```python
from build123d import *

# Parameters (mm, degrees)
SKETCH_1_W          = 60
SKETCH_1_H          = 24
EXTRUDE_1_DEPTH     = 5
SKETCH_2_W          = 31.5
SKETCH_2_H          = 9
SKETCH_2_H_2        = 3
EXTRUDE_2_DEPTH     = 15
SKETCH_3_R          = 1.9
CUT_EXTRUDE_1_DEPTH = 24
SKETCH_4_R          = 4.5
CUT_EXTRUDE_2_DEPTH = 24
FILLET_1_R          = 10
CUT_EXTRUDE_3_DEPTH = 3
SKETCH_7_R          = 1.5
CUT_EXTRUDE_4_DEPTH = 3
CUT_EXTRUDE_5_DEPTH = 6
SKETCH_9_W          = 4.8
SKETCH_9_H          = 12.477545801
CUT_EXTRUDE_6_DEPTH = 3
SKETCH_10_W         = 4.8
SKETCH_10_H         = 29.172350056
CUT_EXTRUDE_7_DEPTH = 3
CHAMFER_1_SIZE      = 3


with BuildPart() as part:
    # Эскиз1 → Бобышка-Вытянуть1 (new body)
    with BuildSketch(Plane(origin=(0, 0, 0), x_dir=(1, 0, 0), z_dir=(0, 1, 0))):
        with Locations((30, 12)):
            Rectangle(SKETCH_1_W, SKETCH_1_H)
    extrude(amount=EXTRUDE_1_DEPTH)

    # Эскиз2 → Бобышка-Вытянуть2 (add)
    with BuildSketch(Plane(origin=(0, 5, 0), x_dir=(1, 0, 0), z_dir=(0, 1, 0))):
        with Locations((30, 4.5)):
            Rectangle(SKETCH_2_W, SKETCH_2_H)
        with Locations((30, 22.5)):
            Rectangle(SKETCH_2_W, SKETCH_2_H_2)
    extrude(amount=EXTRUDE_2_DEPTH)

    # Эскиз3 → Вырез-Вытянуть1 (cut)
    with BuildSketch(Plane.XY):
        with Locations((26.25, 15)):
            Circle(SKETCH_3_R)
    extrude(amount=-CUT_EXTRUDE_1_DEPTH, mode=Mode.SUBTRACT)

    # Эскиз4 → Вырез-Вытянуть2 (cut)
    with BuildSketch(Plane.XZ):
        with Locations(Location((7, -12, 0), (0, 0, 270))):
            Circle(SKETCH_4_R)
        with Locations(Location((53, -12, 0), (0, 0, 270))):
            Circle(SKETCH_4_R)
    extrude(amount=-CUT_EXTRUDE_2_DEPTH, mode=Mode.SUBTRACT)

    # Скругление1
    fillet_1_edges = [part.edges().sort_by_distance(p)[0] for p in [
        (0, 2.5, -24),
        (60, 2.5, -24),
        (60, 2.5, 0),
        (0, 2.5, 0),
    ]]
    fillet(fillet_1_edges, radius=FILLET_1_R)

    # Эскиз5 → Вырез-Вытянуть3 (cut)
    with BuildSketch(Plane(origin=(0, 5, 0), x_dir=(1, 0, 0), z_dir=(0, 1, 0))):
        Polygon((43, 16.732050808), (43, 13.267949192), (46, 11.535898385), (49, 13.267949192), (49, 16.732050808), (46, 18.464101615), align=None)
        Polygon((11, 16.732050808), (11, 13.267949192), (14, 11.535898385), (17, 13.267949192), (17, 16.732050808), (14, 18.464101615), align=None)
    extrude(amount=-CUT_EXTRUDE_3_DEPTH, mode=Mode.SUBTRACT)

    # Эскиз7 → Вырез-Вытянуть4 (cut)
    with BuildSketch(Plane(origin=(0, 2, 0), x_dir=(1, 0, 0), z_dir=(0, 1, 0))):
        with Locations(Location((14, 15, 0), (0, 0, 270))):
            Circle(SKETCH_7_R)
        with Locations(Location((46, 15, 0), (0, 0, 270))):
            Circle(SKETCH_7_R)
    extrude(amount=-CUT_EXTRUDE_4_DEPTH, mode=Mode.SUBTRACT)

    # Эскиз8 → Вырез-Вытянуть5 (cut)
    with BuildSketch(Plane.XY):
        Polygon((27.982050808, 18), (24.517949192, 18), (22.785898385, 15), (24.517949192, 12), (27.982050808, 12), (29.714101615, 15), align=None)
    extrude(amount=-CUT_EXTRUDE_5_DEPTH, mode=Mode.SUBTRACT)

    # Эскиз9 → Вырез-Вытянуть6 (cut)
    with BuildSketch(Plane.ZY.offset(-14.25)):
        with Locations((-4.9, 14.445052705)):
            Rectangle(SKETCH_9_W, SKETCH_9_H)
    extrude(amount=-CUT_EXTRUDE_6_DEPTH, mode=Mode.SUBTRACT)

    # Эскиз10 → Вырез-Вытянуть7 (cut)
    with BuildSketch(Plane(origin=(45.75, 0, 0), x_dir=(0, 0, -1), z_dir=(1, 0, 0))):
        with Locations((4.9, 22.792454832)):
            Rectangle(SKETCH_10_W, SKETCH_10_H)
    extrude(amount=-CUT_EXTRUDE_7_DEPTH, mode=Mode.SUBTRACT)

    # Фаска1
    # the kernel refuses this chamfer: 3 mm, written as the material it takes off along each edge
    with BuildSketch(Plane(origin=(50, 0, -24), x_dir=(0, -0.02749587661058636, 0.9996219169112968), z_dir=(-1, 0, 0))) as chamfer_1_piece_1:
        Polygon((CHAMFER_1_SIZE * 0.999621916911, CHAMFER_1_SIZE * 0.0274958766106), (-CHAMFER_1_SIZE * 0.0274958766106, CHAMFER_1_SIZE * 0.999621916911), (0, 0), align=None)
    extrude(amount=40, mode=Mode.SUBTRACT)
    with BuildSketch(Plane(origin=(0, 0, -14), x_dir=(0.9996219169112968, -0.02749587661058636, 0), z_dir=(0, 0, 1)), Plane(origin=(60, 0, -10), x_dir=(-0.9996219169112968, -0.02749587661058636, 0), z_dir=(0, 0, -1))) as chamfer_1_piece_2:
        Polygon((CHAMFER_1_SIZE * 0.999621916911, CHAMFER_1_SIZE * 0.0274958766106), (-CHAMFER_1_SIZE * 0.0274958766106, CHAMFER_1_SIZE * 0.999621916911), (0, 0), align=None)
    extrude(amount=4, mode=Mode.SUBTRACT)
    with BuildSketch(Plane(origin=(10, 0, 0), x_dir=(0, 0.9996219169112968, 0.027495876610586372), z_dir=(1, 0, 0))) as chamfer_1_piece_3:
        Polygon((CHAMFER_1_SIZE * 0.999621916911, -CHAMFER_1_SIZE * 0.0274958766106), (-CHAMFER_1_SIZE * 0.0274958766106, -CHAMFER_1_SIZE * 0.999621916911), (0, 0), align=None)
    extrude(amount=40, mode=Mode.SUBTRACT)
    with BuildSketch(Plane(origin=(10, 0, -14), x_dir=(-1, 0, 0), z_dir=(0, 0, 1))) as chamfer_1_piece_4:
        Polygon((10 - CHAMFER_1_SIZE, 0), (10, -CHAMFER_1_SIZE), (10, 0), align=None)
    revolve(axis=Axis((10, 0, -14), (0, -1, 0)), revolution_arc=90, mode=Mode.SUBTRACT)
    with BuildSketch(Plane(origin=(10, 0, -10), x_dir=(0, 0, 1), z_dir=(1, 0, 0))) as chamfer_1_piece_5:
        Polygon((10 - CHAMFER_1_SIZE, 0), (10, -CHAMFER_1_SIZE), (10, 0), align=None)
    revolve(axis=Axis((10, 0, -10), (0, -1, 0)), revolution_arc=90, mode=Mode.SUBTRACT)
    with BuildSketch(Plane(origin=(50, 0, -10), x_dir=(0, 0, 1), z_dir=(-1, 0, 0))) as chamfer_1_piece_6:
        Polygon((10 - CHAMFER_1_SIZE, 0), (10, CHAMFER_1_SIZE), (10, 0), align=None)
    revolve(axis=Axis((50, 0, -10), (0, 1, 0)), revolution_arc=90, mode=Mode.SUBTRACT)
    with BuildSketch(Plane(origin=(50, 0, -14), x_dir=(1, 0, 0), z_dir=(0, 0, 1))) as chamfer_1_piece_7:
        Polygon((10 - CHAMFER_1_SIZE, 0), (10, CHAMFER_1_SIZE), (10, 0), align=None)
    revolve(axis=Axis((50, 0, -14), (0, 1, 0)), revolution_arc=90, mode=Mode.SUBTRACT)


solid = part.part
```
Source: CAD feature listing. Evaluate the final solid. Frame: model axes, mm. A direction names the side the tool comes from. Coordinates: 2 decimals unless noted, no trailing zeros. Loops run counter-clockwise (first coordinate to the right, second up) from the corner with the lowest first, then second, coordinate; pieces in that order, holes last. Notation, with made-up numbers: (19, -11) -> (41, -11) arc R8 cw to (41, 1) -> close; hole circle Ø2 at (-13.75, 40.25). An arc over 180 degrees is marked (long way). One line per item, written item: value. Start each with the question number.
Q1. Section query C-C, the plane z = -15. Give the number of separate pieces and of enclosed holes in the cut face, and give its area (3 significant figures).
Q2. Mould query, pull axis Y, two halves, no side actions, for faces 1 (the face through (28.86, 16.48, -2.96)), 2 (the face through (44, 8.206, -5)), 3 (the face through (30, 11, 0)). Classes: pulls with the +Y half, pulls with the -Y half, needs draft (parallel to the pull), parting line crosses it, or undercut.
Q3. Section query A-A, the plane x = 26.25. Return the cut outline in (y, z).
Q4. Set-up query: faces 4 (the face through (44, 14, -7.3)), 5 (the face through (17.25, 14, -5)), 6 (the face through (13.3, 2, -13.5)), 7 (the face through (30, 12, -9)). Return all of +Z, -Z, +X, -X, +Y, -Y with unobstructed straight access to the full face (end or side cutting, diameter ignored); none if empty.
Q5. Section query B-B, the plane y = 16. Return the cut outline in (x, z), and give its area (3 significant figures).
Q6. Line query: line 1 along Z through (x, y) = (45.5, 17.75); line 2 along X through (y, z) = (4.5, -17.25); line 3 along Z through (x, y) = (29.5, 12.75). Output: solid intervals per line, ascending.
Q7. Contact query for flat-ended pins moving along their axis: P1, Ø10, axis at y = 14, z = -6.5, coming from the -X side; P2, Ø0.9, axis at x = 15.5, z = -5, coming from the +Y side; P3, Ø3.5, axis at x = 46, z = -15, coming from the +Y side. Output: stop coordinate, or through.
Results:
1. separate pieces: 5
1. enclosed holes: 0
1. area: 175 mm^2
2. face 1: undercut
2. face 2: pulls with the +Y half
2. face 3: needs draft
3. outline: (0, -21) -> (3, -24) -> (13.1, -24) -> (13.1, -21) -> (5, -21) -> (5, -9) -> (13.1, -9) -> (13.1, -6) -> (12, -6) -> (12, 0) -> (3, 0) -> (0, -3) -> close; (16.9, -24) -> (20, -24) -> (20, -21) -> (16.9, -21) -> close; (16.9, -9) -> (20, -9) -> (20, 0) -> (18, 0) -> (18, -6) -> (16.9, -6) -> close
4. face 4: +X, +Y
4. face 5: -X, +Y
4. face 6: +Y
4. face 7: +X, -X, +Y
5. outline: (14.25, -24) -> (24.63, -24) -> (24.63, -21) -> (14.25, -21) -> close; (14.25, -9) -> (24.63, -9) -> (24.63, -6) -> (23.36, -6) -> (23.36, 0) -> (14.25, 0) -> (14.25, -2.5) -> (17.25, -2.5) -> (17.25, -7.3) -> (14.25, -7.3) -> close; (27.87, -24) -> (45.75, -24) -> (45.75, -21) -> (27.87, -21) -> close; (27.87, -9) -> (45.75, -9) -> (45.75, -7.3) -> (42.75, -7.3) -> (42.75, -2.5) -> (45.75, -2.5) -> (45.75, 0) -> (29.14, 0) -> (29.14, -6) -> (27.87, -6) -> close
5. area: 295 mm^2
6. line 1: -24 to -21, -9 to -7.3, -2.5 to 0
6. line 2: 0.54 to 11.9, 16.1 to 43.9, 48.1 to 59.46
6. line 3: -24 to -21, -9 to 0
7. P1: x = 14.25
7. P2: y = 8.21
7. P3: y = 2
